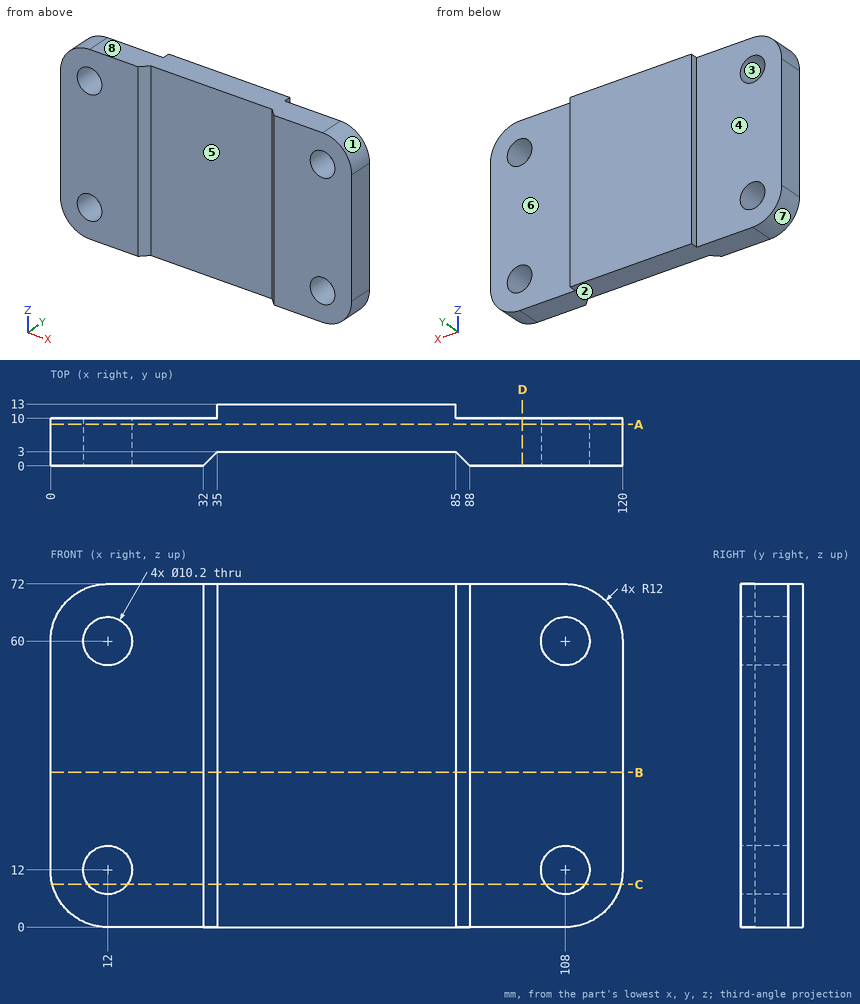
Answer from the drawing. Dimensions are ordinates in mm from the lowest x, y and z of the part. A direction names the side the tool comes from. Round coordinates to 2 decimals unless told otherwise and drop trailing zeros. Loops run counter-clockwise (first coordinate to the right, second up) from the corner with the lowest first, then second, coordinate; pieces in that order, holes last.
(1) Find the intervals of material crossed by L1, parallel to Z at x = 108, y = 7.25; L2, parallel to X at y = 6, z = 12; L3, parallel to X at y = 1.5, z = 61, in increasing order.
Computed values:
L1: z = 0 to 6.9, 17.1 to 54.9, 65.1 to 72
L2: x = 0 to 6.9, 17.1 to 102.9, 113.1 to 120
L3: x = 0.04 to 7, 17 to 33.5, 86.5 to 103, 113 to 119.96
(2) The part is cut by section A-A, the plane y = 8.75. Give the vertices of the cut face in (x, z).
Computed values:
outline: (0, 12) arc R12 ccw to (12, 0) - (108, 0) arc R12 ccw to (120, 12) - (120, 60) arc R12 ccw to (108, 72) - (12, 72) arc R12 ccw to (0, 60) - close; hole circle Ø10.2 at (12, 12); hole circle Ø10.2 at (12, 60); hole circle Ø10.2 at (108, 12); hole circle Ø10.2 at (108, 60)
(3) Each of these flat-tipped pins is pushed along its axis until it touches: P1, Ø10, axis at x = 99, z = 47.5, coming from the +Y side; P2, Ø15, axis at x = 59.5, z = 26.5, coming from the -Y side; P3, Ø1.5, axis at y = 11, z = 39.5, coming from the -X side; P4, Ø6, axis at x = 12, z = 60, coming from the +Y side. Where does it stop, or does it pass through?
Computed values:
P1: stops at y = 10
P2: stops at y = 3
P3: stops at x = 35
P4: passes through
(4) For the marked faces 4, 5, 6, 7 and 8, determine the directions among +Z, -Z, +X, -X, +Y, -Y from which every point of the face is accessible in a straight line to the end or side of a thin tool.
Computed values:
face 4: +Z, -Z, -X, +Y
face 5: +Z, -Z, -Y
face 6: +Z, -Z, +X, +Y
face 7: -Z, -X, +Y, -Y
face 8: +Z, +X, -X, +Y, -Y
(5) The part is cut by section C-C, the plane z = 9. Give the vertices of the cut face in (x, y), and give its area (3 significant figures).
Computed values:
outline: (0.38, 0) - (7.88, 0) - (7.88, 10) - (0.38, 10) - close; (16.12, 0) - (32, 0) - (35, 3) - (85, 3) - (88, 0) - (103.88, 0) - (103.88, 10) - (85, 10) - (85, 13) - (35, 13) - (35, 10) - (16.12, 10) - close; (112.12, 0) - (119.62, 0) - (119.62, 10) - (112.12, 10) - close
area: 1,020 mm2
(6) The mould has two halves that part along X. Classify the marked faces 1, 2 and 3: pulls with the +X half, pulls with the -X half, needs draft (parallel to the pull), parting line crosses it, or undercut.
Computed values:
face 1: pulls with the +X half
face 2: needs draft
face 3: undercut
(7) The part is cut by section D-D, the plane x = 99. Give the vertices of the cut face in (y, z), and give its area (3 significant figures).
Computed values:
outline: (0, 0) - (10, 0) - (10, 72) - (0, 72) - close
area: 720 mm2
(8) The part is cut by section B-B, the plane z = 32.5. Give the vertices of the cut face in (x, y), and give its area (3 significant figures).
Computed values:
outline: (0, 0) - (32, 0) - (35, 3) - (85, 3) - (88, 0) - (120, 0) - (120, 10) - (85, 10) - (85, 13) - (35, 13) - (35, 10) - (0, 10) - close
area: 1,190 mm2
